Autodesk Inventor part; units mm, degrees
ref_plane "工作平面1" through (0, 0, 0) normal (0, 0, 1) x (1, 0, 0)
ref_plane "YZ Plane" through (0, 0, 0) normal (1, 0, 0) x (0, 1, 0)
ref_plane "XZ Plane" through (0, 0, 0) normal (0, 1, 0) x (-1, 0, 0)
ref_plane "工作平面1" through (0, 0, 0) normal (0, 0, 1) x (1, 0, 0)
sketch "草图1" plane through (0, 0, 0) normal (0, 0, 1) x (1, 0, 0)
  circle A0 centre (41.25, -71.4471) radius 5.5
  circle A1 centre (41.25, 71.4471) radius 5.5
  circle A2 centre (82.5, 0) radius 5.5
  circle A3 centre (-82.5, 0) radius 5.5
  circle A4 centre (-41.25, 71.4471) radius 5.5
  circle A5 centre (-41.25, -71.4471) radius 5.5
  circle A6 centre (0, 0) radius 95
  circle A7 centre (0, 0) radius 72.9612
  point P0 (0, 0)
extrude "拉伸1" add sketch "草图1" along normal blind 0.18
properties part number "垫片2"
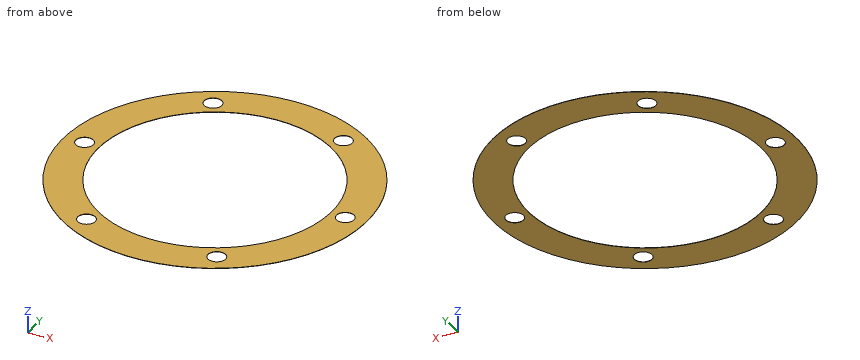
Can you work these out from the model? Positions are in its coordinate system, mm. Give positions to 0.01 mm unless a question says otherwise; leave off trailing zeros. Order: outer loops, then holes, each group sorted by start corner. A loop starts at its lowest first (then second) coordinate and runs counter-clockwise, first axis right, second up. Notation, with made-up numbers: M -4.5,86.5 L 2.5,86.5 A28 cw 2.5,107.5 Z; hole C -14,52 d2. An arc over 180 degrees is marked long. One line per question, with ' | ' between items.
Item 1: Suppose I cut it at B-B, the plane x = 0. Write out the boundary of the cut face in (y, z), then the cut area to 3 significant figures.
Answer block:
outline: M -95,0 L -72.96,0 L -72.96,0.18 L -95,0.18 Z; M 72.96,0 L 95,0 L 95,0.18 L 72.96,0.18 Z | area: 7.93 mm2
Item 2: Suppose I cut it at A-A, the plane y = 0. Write out the boundary of the cut face in (x, z), then the cut area to 3 significant figures.
Answer block:
outline: M -95,0 L -88,0 L -88,0.18 L -95,0.18 Z; M -77,0 L -72.96,0 L -72.96,0.18 L -77,0.18 Z; M 72.96,0 L 77,0 L 77,0.18 L 72.96,0.18 Z; M 88,0 L 95,0 L 95,0.18 L 88,0.18 Z | area: 3.97 mm2
Item 3: Suppose I cut it at C-C, the plane x = -41.25. Write out the boundary of the cut face in (y, z).
Answer block:
outline: M -85.58,0 L -76.95,0 L -76.95,0.18 L -85.58,0.18 Z; M -65.95,0 L -60.18,0 L -60.18,0.18 L -65.95,0.18 Z; M 60.18,0 L 65.95,0 L 65.95,0.18 L 60.18,0.18 Z; M 76.95,0 L 85.58,0 L 85.58,0.18 L 76.95,0.18 Z
Item 4: Suppose I cut it at D-D, the plane z = 0.1. Write out the boundary of the cut face in (x, y).
Answer block:
outline: C 0,0 d190; hole C -82.5,0 d11; hole C 0,0 d145.92; hole C -41.25,-71.45 d11; hole C -41.25,71.45 d11; hole C 41.25,-71.45 d11; hole C 41.25,71.45 d11; hole C 82.5,0 d11
Item 5: Please list where these lines run through material, in increasing order: L1, parallel to Y at x = 41.25, z = 0.1; L2, parallel to Y at x = -39.5, z = 0.1; L3, parallel to Y at x = 0, z = 0.1.
Answer block:
L1: y = -85.58 to -76.95, -65.95 to -60.18, 60.18 to 65.95, 76.95 to 85.58 | L2: y = -86.4 to -76.66, -66.23 to -61.34, 61.34 to 66.23, 76.66 to 86.4 | L3: y = -95 to -72.96, 72.96 to 95
